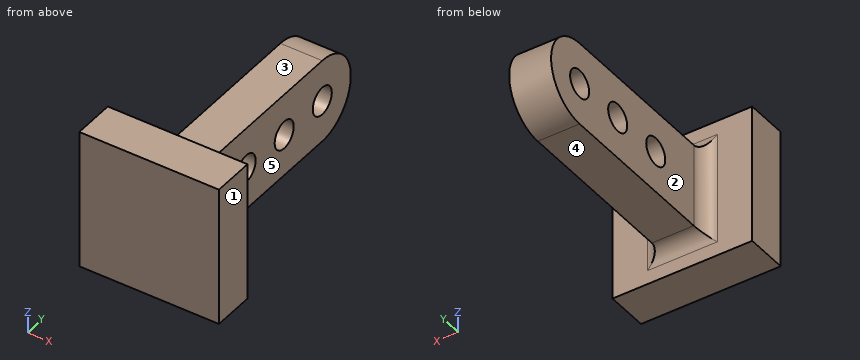
```python
from build123d import *

# Parameters (mm, degrees)
SKETCH1_W           = 10
SKETCH1_H           = 10
BOSS_EXTRUDE1_DEPTH = 3
SKETCH2_R           = 1
BOSS_EXTRUDE2_DEPTH = 1.5
FILLET1_R           = 1


with BuildPart() as part:
    # Sketch1 → Boss-Extrude1 (new body)
    with BuildSketch(Plane(origin=(0, 0, 0), x_dir=(1, 0, 0), z_dir=(0, 1, 0))):
        Rectangle(SKETCH1_W, SKETCH1_H)
    extrude(amount=BOSS_EXTRUDE1_DEPTH)

    # Sketch2 → Boss-Extrude2 (add, symmetric)
    with BuildSketch(Plane(origin=(0, 0, 0), x_dir=(0, 0, -1), z_dir=(1, 0, 0))):
        with BuildLine():
            Line((-3, 3), (-3, 16))
            ThreePointArc((-3, 16), (0, 19), (3, 16))
            Line((3, 16), (3, 3))
            Line((3, 3), (-3, 3))
        make_face()
        with Locations((0, 16)):
            Circle(SKETCH2_R, mode=Mode.SUBTRACT)
        with Locations((0, 12)):
            Circle(SKETCH2_R, mode=Mode.SUBTRACT)
        with Locations((0, 8)):
            Circle(SKETCH2_R, mode=Mode.SUBTRACT)
    extrude(amount=BOSS_EXTRUDE2_DEPTH, both=True)

    # Fillet1
    fillet1_edges = [part.edges().sort_by_distance(p)[0] for p in [
        (1.5, 3, 0),
        (-1.5, 3, 0),
        (0, 3, 3),
        (0, 3, -3),
    ]]
    fillet(fillet1_edges, radius=FILLET1_R)


solid = part.part
```
The model under review builds one solid part; all positions refer to its coordinate system, in mm. Face numbers are marked on the shaded views. A direction names the side the tool comes from. Round coordinates to 2 decimals unless told otherwise and drop trailing zeros. Write each loop counter-clockwise with the first axis right and the second up, starting at its lowest first coordinate (ties: lowest second). Pieces come first, ordered by that corner, then holes.
(1) We need section C-C on x = -1.75. Give the boundary of the cut face in (y, z), and give its area (3 significant figures).
(2) We need section D-D on z = 1.5. Give the boundary of the cut face in (x, y).
(3) Insertion check: pin 1 (1.5 mm diameter, centred on x = -1.5, y = 11, fed in from -Z); pin 2 (3.5 mm diameter, centred on x = 0, y = 8.5, fed in from +Z); pin 3 (2.5 mm diameter, centred on y = 16, z = 0, fed in from +X). Each pin has a flat end and moves straight along its axis. Give the tip position at first contact, or say it passes through.
(4) Wall thickness on L1, parallel to Y at x = 0.6, z = 0; L2, parallel to Y at x = 0.25, z = 0.75; L3, parallel to X at y = 12, z = 2.25: over which ranges is each line inside the solid? List them lowest first.
(5) We need section A-A on y = 8. Give the boundary of the cut face in (x, z), and give its area (3 significant figures).
(6) We need section B-B on z = 0. Give the boundary of the cut face in (x, y), and give its area (3 significant figures).
(7) Machinability: for the marked faces 1, 2, 3, 4 and 5, which of the approach directions +Z, -Z, +X, -X, +Y, -Y give a long, thin tool a straight path to every point of the face, cutting with its end or side? Answer none if there is none.
Findings below:
1. outline: (0, -5) - (3, -5) - (3, -4) arc R1 cw to (3.34, -3.25) - (3.34, 3.25) arc R1 cw to (3, 4) - (3, 5) - (0, 5) - close
1. area: 32.4 mm2
2. outline: (-5, 0) - (5, 0) - (5, 3) - (2.5, 3) arc R1 cw to (1.5, 4) - (1.5, 18.6) - (-1.5, 18.6) - (-1.5, 4) arc R1 cw to (-2.5, 3) - (-5, 3) - close
3. pin 1: stops at z = -3
3. pin 2: stops at z = 3
3. pin 3: stops at x = 1.5
4. L1: y = 0 to 7, 9 to 11, 13 to 15, 17 to 19
4. L2: y = 0 to 7.34, 8.66 to 11.34, 12.66 to 15.34, 16.66 to 18.9
4. L3: x = -1.5 to 1.5
5. outline: (-1.5, -3) - (1.5, -3) - (1.5, -1) - (-1.5, -1) - close; (-1.5, 1) - (1.5, 1) - (1.5, 3) - (-1.5, 3) - close
5. area: 12.0 mm2
6. outline: (-5, 0) - (5, 0) - (5, 3) - (2.5, 3) arc R1 cw to (1.5, 4) - (1.5, 7) - (-1.5, 7) - (-1.5, 4) arc R1 cw to (-2.5, 3) - (-5, 3) - close; (-1.5, 9) - (1.5, 9) - (1.5, 11) - (-1.5, 11) - close; (-1.5, 13) - (1.5, 13) - (1.5, 15) - (-1.5, 15) - close; (-1.5, 17) - (1.5, 17) - (1.5, 19) - (-1.5, 19) - close
6. area: 60.4 mm2
7. face 1: +Z, -Z, +X, +Y, -Y
7. face 2: +Z, -Z, -X, +Y
7. face 3: +Z, +X, -X, +Y
7. face 4: -Z, +X, -X, +Y
7. face 5: +Z, -Z, +X, +Y
